```python
from build123d import *

# Parameters (mm, degrees)
F0_W     = 2.7
F0_H     = 1.5
F0_R     = 3.3
F0_W_2   = 25
F0_H_2   = 17.7
F0_W_3   = 6.5
F0_H_3   = 3
F1_DEPTH = 1.6
F2_R     = 3
F3_SIZE  = 0.25


with BuildPart() as f1:
    # F0 (on Top) → F1 (new body)
    with BuildSketch(Plane.XY):
        Polygon((18, -17.5), (18, 17.5), (12.5, 17.5), (6, 17.5), (-6, 17.5), (-12.5, 17.5), (-18, 17.5), (-18, -17.5), (-12.5, -17.5), (-6, -17.5), (6, -17.5), (12.5, -17.5), align=None)
        with Locations((-5.65, -15.75)):
            Rectangle(F0_W, F0_H, mode=Mode.SUBTRACT)
        with Locations((-5.65, -7.25)):
            Rectangle(F0_W, F0_H, mode=Mode.SUBTRACT)
        with Locations((5.65, -15.75)):
            Rectangle(F0_W, F0_H, mode=Mode.SUBTRACT)
        with Locations((0, -11.5)):
            Circle(F0_R, mode=Mode.SUBTRACT)
        with Locations((5.65, -7.25)):
            Rectangle(F0_W, F0_H, mode=Mode.SUBTRACT)
        with Locations((0, 4.65)):
            Rectangle(F0_W_2, F0_H_2, mode=Mode.SUBTRACT)
        with Locations((9.25, 19)):
            Rectangle(F0_W_3, F0_H_3)
        with Locations((9.25, -19)):
            Rectangle(F0_W_3, F0_H_3)
        with Locations((-9.25, 19)):
            Rectangle(F0_W_3, F0_H_3)
        with Locations((-9.25, -19)):
            Rectangle(F0_W_3, F0_H_3)
    extrude(amount=F1_DEPTH)

    # F2
    f2_edges = [f1.edges().sort_by_distance(p)[0] for p in [
        (-18, 17.5, 0.8),
        (-18, -17.5, 0.8),
        (18, -17.5, 0.8),
        (18, 17.5, 0.8),
        (-12.5, -4.2, 0.8),
        (-12.5, 13.5, 0.8),
        (12.5, 13.5, 0.8),
        (12.5, -4.2, 0.8),
    ]]
    fillet(f2_edges, radius=F2_R)

    # F3
    f3_edges = [f1.edges().sort_by_distance(p)[0] for p in [
        (18, 0, 0),
        (17.12132, -16.62132, 0),
        (17.12132, 16.62132, 0),
        (13.75, -17.5, 0),
        (13.75, 17.5, 0),
        (12.5, -19, 0),
        (12.5, 19, 0),
        (9.25, -20.5, 0),
        (9.25, 20.5, 0),
        (6, -19, 0),
        (6, 19, 0),
        (0, -17.5, 0),
        (0, 17.5, 0),
        (-6, -19, 0),
        (-6, 19, 0),
        (-9.25, -20.5, 0),
        (-9.25, 20.5, 0),
        (-12.5, -19, 0),
        (-12.5, 19, 0),
        (-13.75, -17.5, 0),
        (-13.75, 17.5, 0),
        (-17.12132, -16.62132, 0),
        (-17.12132, 16.62132, 0),
        (-18, 0, 0),
        (-7, -15.75, 0),
        (-5.65, -15, 0),
        (-4.3, -15.75, 0),
        (-5.65, -16.5, 0),
        (-4.3, -7.25, 0),
        (-5.65, -8, 0),
        (-7, -7.25, 0),
        (-5.65, -6.5, 0),
        (4.3, -15.75, 0),
        (5.65, -15, 0),
        (7, -15.75, 0),
        (5.65, -16.5, 0),
        (-3.3, -11.5, 0),
        (5.65, -8, 0),
        (4.3, -7.25, 0),
        (5.65, -6.5, 0),
        (7, -7.25, 0),
        (-12.5, 4.65, 0),
        (-11.62132, -3.32132, 0),
        (-11.62132, 12.62132, 0),
        (0, -4.2, 0),
        (0, 13.5, 0),
        (11.62132, -3.32132, 0),
        (11.62132, 12.62132, 0),
        (12.5, 4.65, 0),
        (-7, -7.25, 1.6),
        (-5.65, -6.5, 1.6),
        (-4.3, -7.25, 1.6),
        (-5.65, -8, 1.6),
        (-5.65, -15, 1.6),
        (-7, -15.75, 1.6),
        (-5.65, -16.5, 1.6),
        (-4.3, -15.75, 1.6),
        (4.3, -7.25, 1.6),
        (5.65, -6.5, 1.6),
        (7, -7.25, 1.6),
        (5.65, -8, 1.6),
        (5.65, -15, 1.6),
        (4.3, -15.75, 1.6),
        (5.65, -16.5, 1.6),
        (7, -15.75, 1.6),
    ]]
    chamfer(f3_edges, length=F3_SIZE)


solid = f1.part
```
Here's how the part is built. I have some questions about the finished solid (model axes, mm). A direction names the side the tool comes from. Coordinates: 2 decimals unless noted, no trailing zeros. Loops run counter-clockwise (first coordinate to the right, second up) from the corner with the lowest first, then second, coordinate; pieces in that order, holes last. Notation, with made-up numbers: (39.25, 72) -> (47.25, 72) arc R19 ccw to (47.25, 82) -> close; hole circle Ø5 at (-3.75, -13.75). An arc over 180 degrees is marked (long way). Return JSON: item names as keys, results as strings.
1) If we section it at D-D, the plane y = 2: Write out the boundary of the cut face in (x, z), then the cut area to 3 significant figures.
Results below:
{"outline": "(-18, 0.25) -> (-17.75, 0) -> (-12.75, 0) -> (-12.5, 0.25) -> (-12.5, 1.6) -> (-18, 1.6) -> close; (12.5, 0.25) -> (12.75, 0) -> (17.75, 0) -> (18, 0.25) -> (18, 1.6) -> (12.5, 1.6) -> close", "area": "17.5 mm²"}
2) If we section it at A-A, the plane y = -11.5: Write out the boundary of the cut face in (x, z).
Results below:
{"outline": "(-18, 0.25) -> (-17.75, 0) -> (-3.55, 0) -> (-3.3, 0.25) -> (-3.3, 1.6) -> (-18, 1.6) -> close; (3.3, 0.25) -> (3.55, 0) -> (17.75, 0) -> (18, 0.25) -> (18, 1.6) -> (3.3, 1.6) -> close"}
3) Will these pins go through, and if not, where does the flat tip stop? pin 1 (6 mm diameter, centred on x = 10, y = 1, fed in from +Z); pin 2 (0.7 mm diameter, centred on x = 2.5, z = 1, fed in from -Y).
Results below:
{"pin 1": "z = 1.6", "pin 2": "y = -17.5"}
4) For faces 1 (the face through (11.6, 12.64, 0.93)), 2 (the face through (6, 19, 1)), 3 (the face through (-12.5, 19, 1)), which set-ups out of +Z, -Z, +X, -X, +Y, -Y let a thin tool reach every point of the face, with its end or its side?
Results below:
{"face 1": "+Z, -Z", "face 2": "+Z, -Z, +Y", "face 3": "+Z, -Z, -X, +Y"}
5) If we section it at C-C, the plane x = -13.5: Write out the boundary of the cut face in (y, z), then the cut area to 3 significant figures.
Results below:
{"outline": "(-17.5, 0.25) -> (-17.25, 0) -> (17.25, 0) -> (17.5, 0.25) -> (17.5, 1.6) -> (-17.5, 1.6) -> close", "area": "55.9 mm²"}
6) If we section it at B-B, the plane x = 0: Write out the boundary of the cut face in (y, z).
Results below:
{"outline": "(-17.5, 0.25) -> (-17.25, 0) -> (-15.05, 0) -> (-14.8, 0.25) -> (-14.8, 1.6) -> (-17.5, 1.6) -> close; (-8.2, 0.25) -> (-7.95, 0) -> (-4.45, 0) -> (-4.2, 0.25) -> (-4.2, 1.6) -> (-8.2, 1.6) -> close; (13.5, 0.25) -> (13.75, 0) -> (17.25, 0) -> (17.5, 0.25) -> (17.5, 1.6) -> (13.5, 1.6) -> close"}
7) Thinking about a two-plate mould opening in X: for faces 4 (the face through (12.5, 19, 1)), 5 (the face through (7, -7, 1)), 6 (the face through (-7, -16, 1)), 7 (the face through (-14, 17.5, 1)), which applies, +X half, -X half, draft (parallel to the pull), parting line (faces both ways), or undercut?
Results below:
{"face 4": "+X half", "face 5": "undercut", "face 6": "undercut", "face 7": "draft"}
8) I need wall thicknesses on line 1 (X direction, y = -7.5, z = 0.7); line 2 (Y direction, x = 0, z = 1.25); line 3 (X direction, y = -1, z = 0.6). Which ranges of each line are inside material? Lowest first, please. Write a range as from..to.
Results below:
{"line 1": "-18..-7, -4.3..4.3, 7..18", "line 2": "-17.5..-14.8, -8.2..-4.2, 13.5..17.5", "line 3": "-18..-12.5, 12.5..18"}
